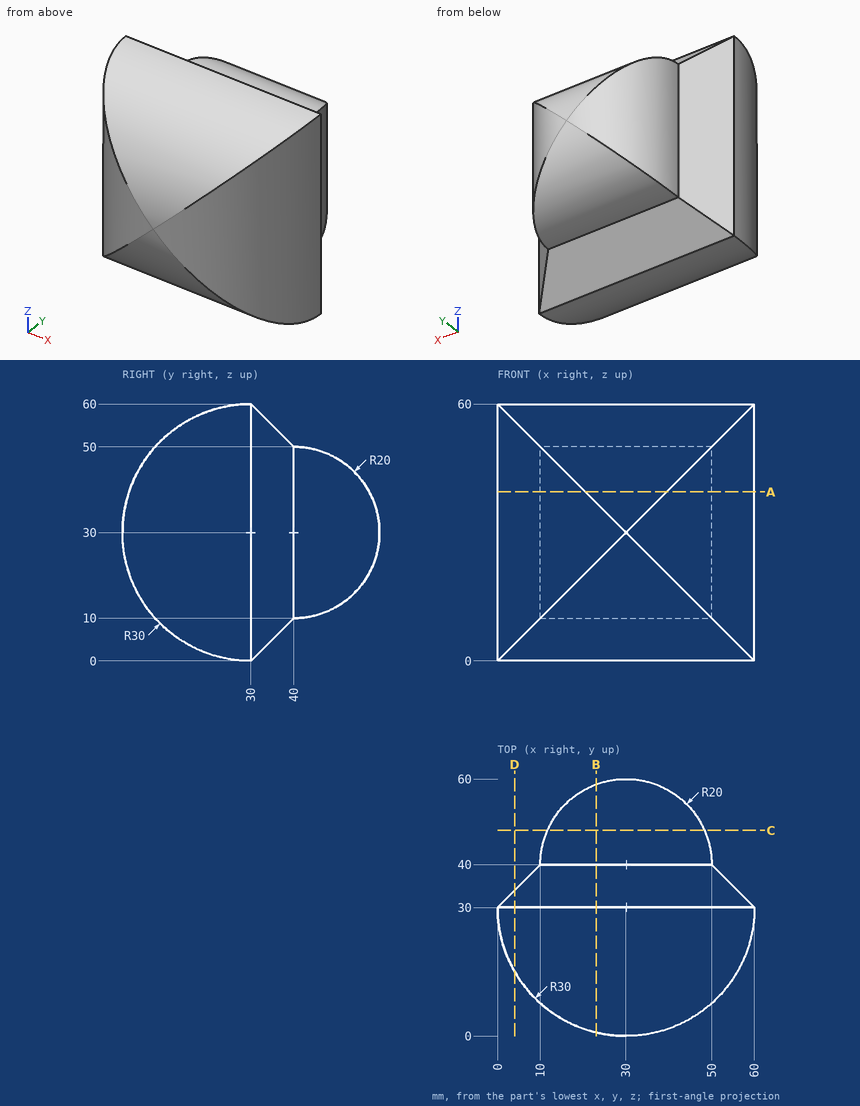
Check sheet for the drawn part. Datum: minimum x, y, z corner. Units: mm. Round coordinates to 2 decimals unless told otherwise and drop trailing zeros. Order: outer loops, then holes, each group sorted by start corner. A loop starts at its lowest first (then second) coordinate and runs counter-clockwise, first axis right, second up. Notation, with made-up numbers: (50, -14) - (92, -14) arc R15 ccw to (92, -10) - close; hole circle Ø7 at (0, 57). An arc over 180 degrees is marked (long way). Use a Markdown table: item, result. Add a question column.
(1) Sectioned sample at D-D, the plane x = 4. Enter the section's corners in (y, z).
(2) Sectioned sample at A-A, the plane z = 39.5. Enter the section's corners in (x, y).
(3) Sectioned sample at C-C, the plane y = 48. Enter the section's corners in (x, z).
(4) Material ranges on line 1 along X through (y, z) = (20.5, 20); line 2 along Z through (x, y) = (18, 45); line 3 along Y through (x, z) = (54, 55), recorded low to high. Write a range as [from, to].
(5) Depth check by flat-ended pin: pin 1 (2 mm diameter, centred on x = 11, z = 45, fed in from -Y); pin 2 (8 mm diameter, centred on y = 37.5, z = 53.5, fed in from +X); pin 3 (1 mm diameter, centred on x = 23, z = 25, fed in from -Y). Enter the tip coordinate at first touch or a pass-through.
(6) Sectioned sample at B-B, the plane x = 23. Enter the section's corners in (y, z) (3 decimals), and give its area (3 significant figures).
Answers below:
| question | item | result |
|---|---|---|
| 1 | outline | (15.03, 4) arc R30 ccw to (30, 0) - (34, 4) - (34, 56) - (30, 60) arc R30 ccw to (15.03, 56) - close |
| 2 | outline | (0, 30) arc R30 ccw to (20.5, 1.54) - (39.5, 1.54) arc R30 ccw to (60, 30) - (50, 40) arc R20 ccw to (39.5, 57.6) - (20.5, 57.6) arc R20 ccw to (10, 40) - close |
| 3 | outline | (11.67, 11.67) - (48.33, 11.67) - (48.33, 48.33) - (11.67, 48.33) - close |
| 4 | line 1 | [1.54, 58.46] |
| 4 | line 2 | [10.64, 49.36] |
| 4 | line 3 | [13.42, 35] |
| 5 | pin 1 | y = 6 |
| 5 | pin 2 | x = 56.5 |
| 5 | pin 3 | y = 0.71 |
| 6 | outline | (0.828, 23) arc R30 ccw to (30, 0) - (40, 10) arc R20 ccw to (58.735, 23) - (58.735, 37) arc R20 ccw to (40, 50) - (30, 60) arc R30 ccw to (0.828, 37) - close |
| 6 | area | 2,520 mm² |
